from build123d import *

# Parameters (mm, degrees)
SKETCH1_R           = 2.0193
SKETCH1_R_2         = 3.3782
BOSS_EXTRUDE1_DEPTH = 6.35
BOSS_EXTRUDE2_START = 120.65
BOSS_EXTRUDE2_DEPTH = 120.65
BOSS_EXTRUDE3_REACH = 145.827
SKETCH6_R           = 3.3782
BOSS_EXTRUDE4_DEPTH = 6.35
FILLET2_R           = 3.175
CHAMFER1_SIZE       = 4.826


with BuildPart() as part:
    # Sketch1 → Boss-Extrude1 (new body)
    with BuildSketch(Plane(origin=(0, 0, 0), x_dir=(0, 0, -1), z_dir=(1, 0, 0))):
        with BuildLine():
            Line((19.857637877, 39.149224239), (42.164, 28.956))
            Line((42.164, 28.956), (42.164, 14.4653))
            Line((42.164, 14.4653), (46.99, 14.4653))
            Line((46.99, 14.4653), (46.99, 77.089))
            Line((46.99, 77.089), (9.62025, 77.089))
            ThreePointArc((9.62025, 77.089), (5.201472483, 76.745277517), (0.889, 75.722379195))
            Line((0.889, 75.722379195), (0.889, 48.514))
            ThreePointArc((0.889, 48.514), (3.422551022, 42.363938704), (9.552880645, 39.783009911))
            Line((9.552880645, 39.783009911), (17.267409525, 39.723483692))
            ThreePointArc((17.267409525, 39.723483692), (18.59285001, 39.573142424), (19.857637877, 39.149224239))
        make_face()
        with Locations((9.62025, 48.514)):
            Circle(SKETCH1_R, mode=Mode.SUBTRACT)
        with Locations((37.4015, 52.0954)):
            Circle(SKETCH1_R_2, mode=Mode.SUBTRACT)
    extrude(amount=-BOSS_EXTRUDE1_DEPTH)

    # Sketch2 → Boss-Extrude2 (add)
    with BuildSketch(Plane(origin=(0, 0, 0), x_dir=(0, 0, -1), z_dir=(1, 0, 0)).offset(BOSS_EXTRUDE2_START)):
        with BuildLine():
            Line((42.164, 35.93758433), (22.496862123, 44.924775761))
            ThreePointArc((22.496862123, 44.924775761), (18.289474239, 43.356612123), (19.857637877, 39.149224239))
            Line((19.857637877, 39.149224239), (42.164, 28.956))
            Line((42.164, 28.956), (42.164, 14.4653))
            Line((42.164, 14.4653), (46.99, 14.4653))
            Line((46.99, 14.4653), (46.99, 77.089))
            Line((46.99, 77.089), (9.62025, 77.089))
            ThreePointArc((9.62025, 77.089), (5.201472483, 76.745277517), (0.889, 75.722379195))
            Line((0.889, 75.722379195), (0.889, 68.952099188))
            ThreePointArc((0.889, 68.952099188), (5.164137875, 70.287692607), (9.62025, 70.739))
            Line((9.62025, 70.739), (42.164, 70.739))
            Line((42.164, 70.739), (42.164, 35.93758433))
        make_face()
    extrude(amount=-BOSS_EXTRUDE2_DEPTH)

    # Boss-Extrude3: up to this plane
    boss_extrude3_end = Plane(origin=(-6.35, 39.893111336, -18.2297511), z_dir=(0, -0.909535672675175, 0.41562586557060793))
    # Sketch5 → Boss-Extrude3 (add, up to the surface)
    with BuildSketch(Plane.XZ.offset(-14.4653), mode=Mode.PRIVATE) as boss_extrude3_sk1:
        Polygon((-3.858864353, -42.164), (8.841135647, -42.164), (6.8e-08, -37.059567994), (-6.35, -37.059567994), (-6.35, -40.725742164), align=None)
    boss_extrude3_tool1 = split(extrude(boss_extrude3_sk1.sketch, amount=-BOSS_EXTRUDE3_REACH, mode=Mode.PRIVATE), bisect_by=boss_extrude3_end, keep=Keep.BOTH, mode=Mode.PRIVATE)
    add(boss_extrude3_tool1.solids().sort_by_distance((-0.498721, 14.4653, -39.902897))[0])
    # Sketch5 → Boss-Extrude3 (add, up to the surface)
    with BuildSketch(Plane.XZ.offset(-14.4653), mode=Mode.PRIVATE) as boss_extrude3_sk2:
        Polygon((-6.35, -42.164), (-3.858864353, -42.164), (-6.35, -40.725742164), align=None)
    boss_extrude3_tool2 = split(extrude(boss_extrude3_sk2.sketch, amount=-BOSS_EXTRUDE3_REACH, mode=Mode.PRIVATE), bisect_by=boss_extrude3_end, keep=Keep.BOTH, mode=Mode.PRIVATE)
    add(boss_extrude3_tool2.solids().sort_by_distance((-5.519621, 14.4653, -41.684581))[0])

    # Sketch6 → Boss-Extrude4 (add)
    with BuildSketch(Plane.ZY.offset(6.35)):
        with BuildLine():
            Line((-26.918328061, 86.341628061), (-36.170956121, 77.089))
            Line((-36.170956121, 77.089), (-16.0782, 77.089))
            Line((-16.0782, 77.089), (-16.0782, 81.8515))
            ThreePointArc((-16.0782, 81.8515), (-19.998160204, 87.718135031), (-26.918328061, 86.341628061))
        make_face()
        with Locations((-22.4282, 81.8515)):
            Circle(SKETCH6_R, mode=Mode.SUBTRACT)
    extrude(amount=-BOSS_EXTRUDE4_DEPTH)

    # Fillet2
    fillet2_edges = [part.edges().sort_by_distance(p)[0] for p in [
        (60.325, 35.93758433, -42.164),
        (60.325, 70.739, -42.164),
        (64.745567823, 28.956, -42.164),
        (-3.174999966, 31.288546193, -37.059567994),
        (8.841135647, 21.71065, -42.164),
        (4.420567858, 30.122273097, -39.611783997),
        (-3.175, 77.089, -16.0782),
        (-3.175, 77.089, -36.170956121),
    ]]
    fillet(fillet2_edges, radius=FILLET2_R)

    # Mirror1: part across plane


with BuildPart() as part_1:
    add(part.part)
    add(part.part.mirror(Plane(origin=(120.65, 0, 0), x_dir=(0, 0, 1), z_dir=(1, 0, 0))))

    # Chamfer1
    chamfer1_edges = [part_1.edges().sort_by_distance(p)[0] for p in [
        (247.65, 45.77715, -46.99),
        (-6.35, 45.77715, -46.99),
    ]]
    chamfer(chamfer1_edges, length=CHAMFER1_SIZE)


solid = part_1.part
Check sheet for the modelled part. Datum: model origin and axes. Units: mm. A direction names the side the tool comes from. Coordinates: 2 decimals unless noted, no trailing zeros. Loops run counter-clockwise (first coordinate to the right, second up) from the corner with the lowest first, then second, coordinate; pieces in that order, holes last. Notation, with made-up numbers: (-9.5, 7.5) -> (47.5, 7.5) arc R16 ccw to (47.5, 32.5) -> close; hole circle Ø2 at (27, 28). An arc over 180 degrees is marked (long way). Write item = value, one per line. Start each with the question number.
1. Tool access check on faces 1 (the cylindrical face through (-3.13, 42.43, -3.36)), 2 (the flat face through (119, 70.739, -24)), 3 (the flat face through (4.109, 21.658, -39.432)). Record the directions out of +Z, -Z, +X, -X, +Y, -Y that give a thin tool (end or side, any length) a straight path to the whole face; none if there is none.
2. Depth check by flat-ended pin: P1, Ø5.5, axis at y = 52.1, z = -37.4, coming from the +X side; P2, Ø1.3, axis at x = 244.5, y = 81, coming from the +Z side; P3, Ø1.7, axis at x = -3, y = 80.5, coming from the +Z side; P4, Ø10, axis at x = 157.5, z = -12.5, coming from the -Y side. Enter the tip coordinate at first touch or a pass-through.
3. Section check B-B on y = 61.5. Record the cut outline in (x, z).
4. Section check D-D on y = 19. Record the cut outline in (x, z) (3 decimals), then the cut area to 3 significant figures.
5. Section check A-A on z = -29.5. Record the cut outline in (x, y).
6. Draft check along Z on faces 4 (the flat face through (-3.903, 45.339, -44.611)), 5 (the flat face through (244, 22, -37.06)), 6 (the flat face through (241.3, 84, -25.4)), 7 (the flat face through (118.96, 41.41, -30.19)). Enter one of: released by +Z, released by -Z, zero draft, split by the parting line, or undercut.
7. Material ranges on line 1 (X direction, y = 61.5, z = -17.5); line 2 (Y direction, x = 22, z = -22.5); line 3 (Z direction, x = 163.5, y = 59.5), recorded low to high.
8. Section check C-C on x = 89. Record the cut outline in (y, z) (3 decimals), then the cut area to 3 significant figures.
Responses:
q1.face_1 = +Z, +X, -X, -Y
q1.face_2 = none
q1.face_3 = +Z, -Y
q2.P1 = through
q2.P2 = -16.08
q2.P3 = -16.02
q2.P4 = 70.64
q3.outline = (-6.35, -42.16) -> (-1.52, -46.99) -> (242.82, -46.99) -> (247.65, -42.16) -> (247.65, -0.89) -> (241.3, -0.89) -> (241.3, -42.16) -> (0, -42.16) -> (0, -0.89) -> (-6.35, -0.89) -> close
q4.outline = (-6.35, -42.164) -> (-1.524, -46.99) -> (242.824, -46.99) -> (247.65, -42.164) -> (247.65, -37.06) -> (241.3, -37.06) -> (233.196, -41.739) arc R3.175 cw to (231.608, -42.164) -> (9.692, -42.164) arc R3.175 cw to (8.104, -41.739) -> (0, -37.06) -> (-6.35, -37.06) -> close
q4.area = 1,310 mm2
q5.outline = (-6.35, 34.74) -> (247.65, 34.74) -> (247.65, 83.76) -> (241.3, 83.76) -> (241.3, 77.09) -> (0, 77.09) -> (0, 83.76) -> (-6.35, 83.76) -> close; hole (0, 41.72) -> (241.3, 41.72) -> (241.3, 70.74) -> (0, 70.74) -> close
q6.face_4 = released by -Z
q6.face_5 = released by +Z
q6.face_6 = zero draft
q6.face_7 = undercut
q7.line_1 = -6.35 to 0, 241.3 to 247.65
q7.line_2 = 37.94 to 44.92, 70.74 to 77.09
q7.line_3 = -46.99 to -42.16
q8.outline = (14.465, -46.99) -> (77.089, -46.99) -> (77.089, -9.62) arc R28.575 ccw to (75.722, -0.889) -> (68.952, -0.889) arc R22.225 cw to (70.739, -9.62) -> (70.739, -38.989) arc R3.175 cw to (67.564, -42.164) -> (40.879, -42.164) arc R3.175 cw to (37.991, -37.669) -> (44.925, -22.497) arc R3.175 ccw to (39.149, -19.858) -> (29.804, -40.309) arc R3.175 cw to (26.916, -42.164) -> (14.465, -42.164) -> close
q8.area = 736 mm2
